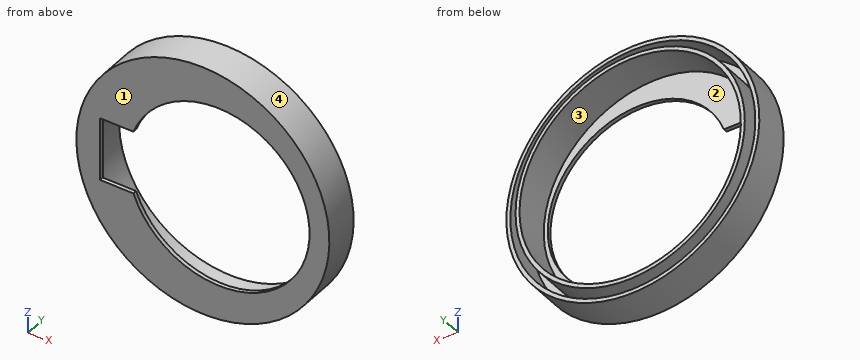
```python
from build123d import *

# Parameters (mm, degrees)
SKETCH1_R           = 16
BOSS_EXTRUDE1_DEPTH = 0.5
SKETCH2_R           = 11.5
CUT_EXTRUDE1_DEPTH  = 0.5
SKETCH3_W           = 15
SKETCH3_H           = 8
CUT_EXTRUDE4_DEPTH  = 2.5
SKETCH4_R           = 16
SKETCH4_R_2         = 15.5
BOSS_EXTRUDE2_DEPTH = 4.5
SKETCH5_R           = 14.5
SKETCH5_R_2         = 14
BOSS_EXTRUDE3_DEPTH = 4.5


with BuildPart() as part:
    # Sketch1 → Boss-Extrude1 (new body)
    with BuildSketch(Plane(origin=(0, 0, 0), x_dir=(1, 0, 0), z_dir=(0, 1, 0))):
        with Locations(Location((0, 0, 0), (0, 0, 270))):
            Circle(SKETCH1_R)
    extrude(amount=BOSS_EXTRUDE1_DEPTH)

    # Sketch2 → Cut-Extrude1 (cut)
    with BuildSketch(Plane(origin=(0, 0.5, 0), x_dir=(1, 0, 0), z_dir=(0, 1, 0))):
        with Locations(Location((2, 0, 0), (0, 0, 270))):
            Circle(SKETCH2_R)
    extrude(amount=-CUT_EXTRUDE1_DEPTH, mode=Mode.SUBTRACT)

    # Sketch3 → Cut-Extrude4 (cut)
    with BuildSketch(Plane(origin=(0, 0, 0), x_dir=(1, 0, 0), z_dir=(0, 1, 0))):
        with Locations((-5.5, 0)):
            Rectangle(SKETCH3_W, SKETCH3_H)
    extrude(amount=CUT_EXTRUDE4_DEPTH, mode=Mode.SUBTRACT)

    # Sketch4 → Boss-Extrude2 (add)
    with BuildSketch(Plane(origin=(0, 0, 0), x_dir=(1, 0, 0), z_dir=(0, 1, 0))):
        with Locations(Location((0, 0, 0), (0, 0, 270))):
            Circle(SKETCH4_R)
        with Locations(Location((0, 0, 0), (0, 0, 270))):
            Circle(SKETCH4_R_2, mode=Mode.SUBTRACT)
    extrude(amount=BOSS_EXTRUDE2_DEPTH)

    # Sketch5 → Boss-Extrude3 (add)
    with BuildSketch(Plane(origin=(0, 0.5, 0), x_dir=(1, 0, 0), z_dir=(0, 1, 0))):
        with Locations(Location((0, 0, 0), (0, 0, 270))):
            Circle(SKETCH5_R)
        with Locations(Location((0, 0, 0), (0, 0, 270))):
            Circle(SKETCH5_R_2, mode=Mode.SUBTRACT)
    extrude(amount=BOSS_EXTRUDE3_DEPTH)


solid = part.part
```
Geometry: final body of the model. Coordinates: model frame, mm. Face numbers are marked on the shaded views. Round coordinates to 2 decimals unless told otherwise and drop trailing zeros. Order: outer loops, then holes, each group sorted by start corner. A loop starts at its lowest first (then second) coordinate and runs counter-clockwise, first axis right, second up. Notation, with made-up numbers: M -25,-40 L 20,-40 A9 cw 20,-26 Z; hole C 17,-11 d6. An arc over 180 degrees is marked long. Use one line per item in the form item = value. Start each with the question number.
Q1. Mould query, pull axis X, two halves, no side actions, for the marked faces 1, 2, 3 and 4. Classes: +X half, -X half, draft (parallel to the pull), parting line (faces both ways), or undercut.
Q2. Cut plane A-A (x = 2). Return loops of the section in (y, z), and give its area (3 significant figures).
Q3. Cut plane C-C (y = 3.5). Return loops of the section in (x, z), and give its area (3 significant figures).
Q4. Pin query (flat end, axial travel): pin 1 Ø0.6 at (x, y) = (-12, 0) entering from -Z; pin 2 Ø14 at (x, z) = (2.5, 6) entering from +Y; pin 3 Ø1 at (x, y) = (1, 3) entering from +Z. Return the tip coordinate at first contact, or that it passes through.
Q5. Material intervals for line 1 (X direction, y = 3.5, z = 0); line 2 (X direction, y = 2.55, z = -5.5); line 3 (X direction, y = 0.4, z = 0), sorted ascending. Write a range as [from, to].
Q6. Cut plane B-B (z = -6). Return loops of the section in (x, y), and give its area (3 significant figures).
Geometry results:
q1.face_1 = draft
q1.face_2 = undercut
q1.face_3 = undercut
q1.face_4 = parting line
q2.outline = M 0,-15.87 L 4.5,-15.87 L 4.5,-15.37 L 0.5,-15.37 L 0.5,-14.36 L 5,-14.36 L 5,-13.86 L 0.5,-13.86 L 0.5,-11.5 L 0,-11.5 Z; M 0,11.5 L 0.5,11.5 L 0.5,13.86 L 5,13.86 L 5,14.36 L 0.5,14.36 L 0.5,15.37 L 4.5,15.37 L 4.5,15.87 L 0,15.87 Z
q2.area = 13.0 mm^2
q3.outline = C 0,0 d32; C 0,0 d29; hole C 0,0 d31; hole C 0,0 d28
q3.area = 94.2 mm^2
q4.pin_1 = -10.91
q4.pin_2 = 0.5
q4.pin_3 = 15.99
q5.line_1 = [-16, -15.5], [-14.5, -14], [14, 14.5], [15.5, 16]
q5.line_2 = [-15.02, -14.49], [-13.42, -12.87], [12.87, 13.42], [14.49, 15.02]
q5.line_3 = [-16, -13], [13.5, 16]
q6.outline = M -14.83,0 L -7.81,0 L -7.81,0.5 L -12.65,0.5 L -12.65,5 L -13.2,5 L -13.2,0.5 L -14.29,0.5 L -14.29,4.5 L -14.83,4.5 Z; M 11.81,0 L 14.83,0 L 14.83,4.5 L 14.29,4.5 L 14.29,0.5 L 13.2,0.5 L 13.2,5 L 12.65,5 L 12.65,0.5 L 11.81,0.5 Z
q6.area = 14.3 mm^2
